Autodesk Inventor part; units mm, degrees
ref_plane "YZ Plane" through (0, 0, 0) normal (1, 0, 0) x (0, 1, 0)
ref_plane "XZ Plane" through (0, 0, 0) normal (0, 1, 0) x (-1, 0, 0)
ref_plane "XY Plane" through (0, 0, 0) normal (0, 0, 1) x (1, 0, 0)
sketch "main" plane through (0, 0, 0) normal (0, 0, 1) x (1, 0, 0)
  circle A0 centre (15.0202, -6.3416) radius 2.1844
  circle A1 centre (37.0172, 6.3584) radius 2.1844
  arc A2 (40.1922, 0.8591) -> (33.8536, 11.8642) centre (37.0172, 6.3584) ccw
  line L0 (-44.2105, -18.3536) -> (5.2134, -18.3536)
  line L1 (40.1922, 0.8591) -> (8.3884, -17.5028)
  circle A3 centre (5.2134, -12.0036) radius 2.0955
  arc A4 (5.2134, -18.3536) -> (8.3884, -17.5028) centre (5.2134, -12.0036) ccw
  line L2 (5.2134, -12.0036) -> (43.3134, -12.0036) construction
  arc A5 (-45.6106, -5.8098) -> (-44.2105, -18.3536) centre (-44.2105, -12.0036) ccw
  line L3 (33.8536, 11.8642) -> (68.8891, 11.8642) construction
  line L4 (-45.6106, -5.8098) -> (35.6171, 12.5521)
  circle A6 centre (-18.8105, -12.0036) radius 2.0955
  circle A7 centre (-44.2105, -12.0036) radius 2.0955
  point P0 (-0.7926, -1.6009)
  dimension "d3" = 12.7
  dimension "d7" = 4.191
  dimension "d8" = 6.35
  dimension "d13" = 25.4
  dimension "d16" = 4.191
sketch "Sketch1" plane through (0, 0, 0) normal (0, 0, 1) x (1, 0, 0)
  circle A0 centre (46.5307, 5.662) radius 2.1844
  circle A1 centre (68.5277, 18.362) radius 2.1844
  arc A2 (71.7027, 12.8627) -> (65.3641, 23.8678) centre (68.5277, 18.362) ccw
  line L0 (-12.7, -6.35) -> (36.7239, -6.35)
  line L1 (71.7027, 12.8627) -> (39.8989, -5.4993)
  circle A3 centre (36.7239, 0) radius 2.0955
  arc A4 (36.7239, -6.35) -> (39.8989, -5.4993) centre (36.7239, 0) ccw
  line L2 (36.7239, 0) -> (74.8239, 0) construction
  arc A5 (-14.1001, 6.1937) -> (-12.7, -6.35) centre (-12.7, 0) ccw
  line L3 (65.3641, 23.8678) -> (100.3996, 23.8678) construction
  line L4 (-14.1001, 6.1937) -> (67.1276, 24.5557)
  circle A6 centre (12.7, 0) radius 2.0955
  circle A7 centre (-12.7, 0) radius 2.0955
  point P0 (0, 0)
extrude "Extrusion1" add sketch "Sketch1" along normal blind 1.5875
equation "\"BendRadius\" = Thickness"
equation "\"BendReliefWidth\" = Thickness"
equation "\"BendReliefDepth\" = 0.5 * Thickness"
equation "\"CornerReliefSize\" = 4 * Thickness"
equation "\"MinimumRemnant\" = 2 * Thickness"
equation "\"TransitionRadius\" = BendRadius"
equation "\"JacobiRadiusSize\" = BendRadius"
equation "\"GapSize\" = Thickness"
properties part number "60 Degree Gusset" material "Acetal Resin, White"
Input: part model. Units: mm. Frame: model coordinates. Coordinates: 2 decimals unless noted, no trailing zeros. Order: outer loops, then holes, each group sorted by start corner. A loop starts at its lowest first (then second) coordinate and runs counter-clockwise, first axis right, second up. Notation, with made-up numbers: M -3,40 L 22,40 A25 cw 22,73 Z; hole C 21.25,-35.5 d7. An arc over 180 degrees is marked long. Write item = value, one per line. Start each with the question number.
(1) Section B-B on x = 12.7. Output: boundary loops of the cut face in (y, z), and give its area (3 significant figures).
(2) Section C-C on z = 1.1. Output: boundary loops of the cut face in (x, y), and give its area (3 significant figures).
(3) Section D-D on y = 11. Output: boundary loops of the cut face in (x, z).
(4) Section A-A on y = 0. Output: boundary loops of the cut face in (x, z).
(5) Line query: line 1 along Y through (x, z) = (47, 1.15); line 2 along Y through (x, z) = (-12.7, 1.25); line 3 along X through (y, z) = (-0.5, 0.95). Output: solid intervals per line, ascending. Write a range as [from, to].
(6) First-contact query: P1, Ø3.5, axis at x = 12.7, y = 0, coming from the +Z side. Flat tip, straight axial feed; report the tip coordinate or a pass-through.
(7) Pull-direction query (X, two-part tool) for faces 1 (the flat face through (25.945, 15.246, 0.783)), 2 (the cylindrical face through (66.8, 19.7, 0.8)), 3 (the flat face through (12, -6.35, 1)), 4 (the cylindrical face through (-10.764, 0.803, 0.783)); classes: released by +X, released by -X, zero draft, split by the parting line, or undercut.
Result set:
q1.outline = M -6.35,0 L -2.1,0 L -2.1,1.59 L -6.35,1.59 Z; M 2.1,0 L 12.25,0 L 12.25,1.59 L 2.1,1.59 Z
q1.area = 22.9 mm²
q2.outline = M -14.1,6.19 A6.35 ccw -12.7,-6.35 L 36.72,-6.35 A6.35 ccw 39.9,-5.5 L 71.7,12.86 A6.35 ccw 67.13,24.56 Z; hole C -12.7,0 d4.19; hole C 12.7,0 d4.19; hole C 36.72,0 d4.19; hole C 46.53,5.66 d4.37; hole C 68.53,18.36 d4.37
q2.area = 1,580 mm²
q3.outline = M 7.16,0 L 68.48,0 L 68.48,1.59 L 7.16,1.59 Z
q4.outline = M -19.05,0 L -14.8,0 L -14.8,1.59 L -19.05,1.59 Z; M -10.6,0 L 10.6,0 L 10.6,1.59 L -10.6,1.59 Z; M 14.8,0 L 34.63,0 L 34.63,1.59 L 14.8,1.59 Z; M 38.82,0 L 49.42,0 L 49.42,1.59 L 38.82,1.59 Z
q5.line_1 = [-1.4, 3.53], [7.8, 20.01]
q5.line_2 = [-6.35, -2.1], [2.1, 6.51]
q5.line_3 = [-19.03, -14.73], [-10.67, 10.67], [14.73, 34.69], [38.76, 48.56]
q6.P1 = through
q7.face_1 = released by -X
q7.face_2 = undercut
q7.face_3 = zero draft
q7.face_4 = undercut
